from build123d import *

# Parameters (mm, degrees)
F0_W     = 80
F0_H     = 30
F1_DEPTH = 37
F2_T     = -2
F4_R     = 1.5
F5_DEPTH = 25
F6_R     = 1.5
F7_DEPTH = 3


with BuildPart() as f1:
    # F0 (on Top) → F1 (new body)
    with BuildSketch(Plane.XY):
        with Locations((1.579888, 0)):
            Rectangle(F0_W, F0_H)
    extrude(amount=F1_DEPTH)

    # F2
    f2_openings = [f1.faces().sort_by_distance(p)[0] for p in [
        (1.579888, 0, 37),
    ]]
    offset(amount=F2_T, openings=f2_openings)

    # F4 (on face) → F5 (cut)
    with BuildSketch(Plane.YZ.offset(41.579888)):
        with Locations((0, 14)):
            Circle(F4_R)
    extrude(amount=-F5_DEPTH, mode=Mode.SUBTRACT)

    # F6 (on face) → F7 (cut)
    with BuildSketch(Plane(origin=(-38.420112, 0, 0), x_dir=(0, -1, 0), z_dir=(-1, 0, 0))):
        with Locations((0, 14)):
            Circle(F6_R)
    extrude(amount=-F7_DEPTH, mode=Mode.SUBTRACT)


solid = f1.part
Geometry check sheet. Reference: the model listing, model coordinates, mm. A direction names the side the tool comes from. Give positions to 0.01 mm unless a question says otherwise; leave off trailing zeros. Loops run counter-clockwise (first coordinate to the right, second up) from the corner with the lowest first, then second, coordinate; pieces in that order, holes last.
(1) Section check D-D on x = -18.5. Record the cut outline in (y, z), then the cut area to 3 significant figures.
From the geometry:
outline: (-15, 0) - (15, 0) - (15, 37) - (13, 37) - (13, 2) - (-13, 2) - (-13, 37) - (-15, 37) - close
area: 200 mm2
(2) Section check A-A on z = 14. Record the cut outline in (x, y).
From the geometry:
outline: (-38.42, -15) - (41.58, -15) - (41.58, -1.5) - (39.58, -1.5) - (39.58, -13) - (-36.42, -13) - (-36.42, -1.5) - (-38.42, -1.5) - close; (-38.42, 1.5) - (-36.42, 1.5) - (-36.42, 13) - (39.58, 13) - (39.58, 1.5) - (41.58, 1.5) - (41.58, 15) - (-38.42, 15) - close
(3) Section check B-B on y = 0. Record the cut outline in (x, z).
From the geometry:
outline: (-38.42, 0) - (41.58, 0) - (41.58, 12.5) - (39.58, 12.5) - (39.58, 2) - (-36.42, 2) - (-36.42, 12.5) - (-38.42, 12.5) - close; (-38.42, 15.5) - (-36.42, 15.5) - (-36.42, 37) - (-38.42, 37) - close; (39.58, 15.5) - (41.58, 15.5) - (41.58, 37) - (39.58, 37) - close
(4) Set-up check for faces 1 (the flat face through (-36.42, 0, 19)), 2 (the flat face through (1, -15, 18)): record each of +Z, -Z, +X, -X, +Y, -Y from which the full face is reachable in a straight line by a thin tool's end or side.
From the geometry:
face 1: +Z
face 2: +Z, -Z, +X, -X, -Y
(5) Depth check by flat-ended pin: pin 1 Ø2 at (x, y) = (23.5, 11.5) entering from +Z; pin 2 Ø1.8 at (y, z) = (0, 14) entering from +X. Enter the tip coordinate at first touch or a pass-through.
From the geometry:
pin 1: stops at z = 2
pin 2: passes through
(6) Release check for a two-part mould opening along Y. For faces 3 (the flat face through (1, 15, 18)), 4 (the flat face through (1, 0, 0)), 5 (the flat face through (39.58, 0, 19)) record: released by +Y, released by -Y, zero draft, split by the parting line, or undercut.
From the geometry:
face 3: released by +Y
face 4: zero draft
face 5: undercut
(7) Thickness scan on L1, parallel to Y at x = 33.5, z = 33.5; L2, parallel to X at y = -10, z = 14.5; L3, parallel to Z at x = 41, y = 0. Record the ranges inside material, lowest first.
From the geometry:
L1: y = -15 to -13, 13 to 15
L2: x = -38.42 to -36.42, 39.58 to 41.58
L3: z = 0 to 12.5, 15.5 to 37
(8) Section check C-C on z = 30. Record the cut outline in (x, y).
From the geometry:
outline: (-38.42, -15) - (41.58, -15) - (41.58, 15) - (-38.42, 15) - close; hole (-36.42, -13) - (39.58, -13) - (39.58, 13) - (-36.42, 13) - close
